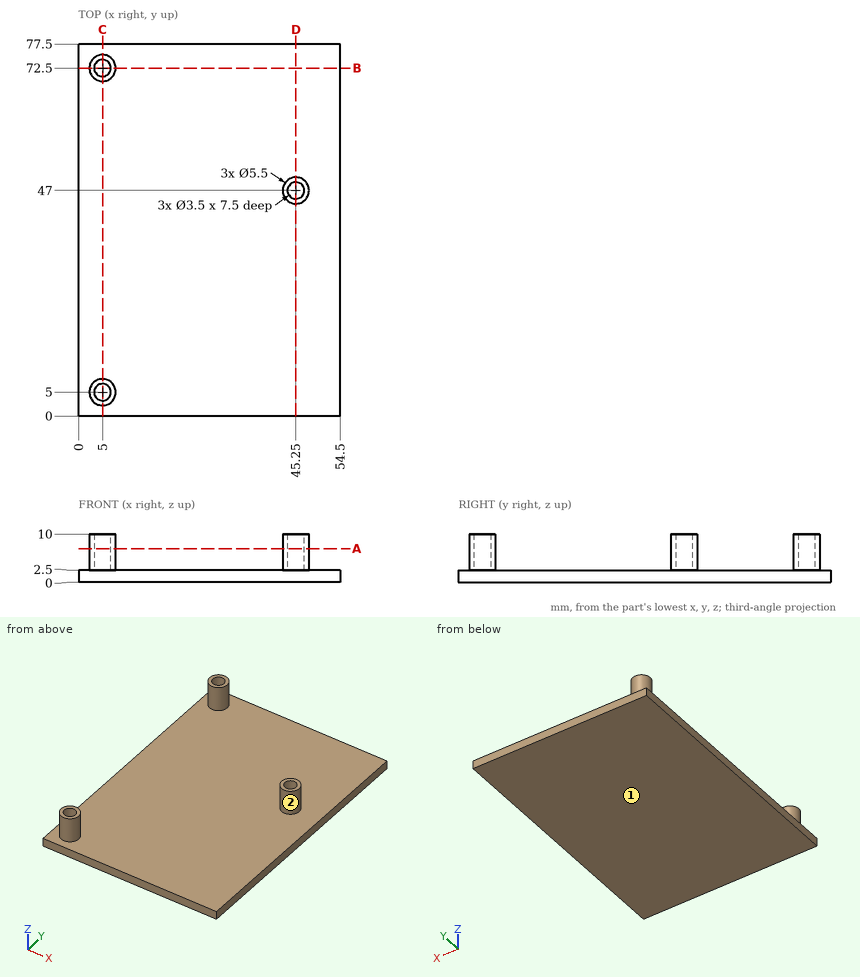
Geometry check sheet. Reference: drawing and pictorial views, mm from the part's lowest x, y, z. A direction names the side the tool comes from. Coordinates: 2 decimals unless noted, no trailing zeros. Write each loop counter-clockwise with the first axis right and the second up, starting at its lowest first coordinate (ties: lowest second). Pieces come first, ordered by that corner, then holes. Notation, with made-up numbers: (-12, 65) -> (12, 65) arc R19 cw to (12, 72) -> close; hole circle Ø10 at (1.5, -6.5). An arc over 180 degrees is marked (long way). Use a Markdown table: item, result.
1. Sectioned sample at A-A (z = 7). Enter the section's corners in (x, y).
Reported:
| item | result |
|---|---|
| outline | circle Ø5.5 at (5, 5); circle Ø5.5 at (5, 72.5); circle Ø5.5 at (45.25, 47); hole circle Ø3.5 at (5, 5); hole circle Ø3.5 at (5, 72.5); hole circle Ø3.5 at (45.25, 47) |
2. Sectioned sample at C-C (x = 5). Enter the section's corners in (y, z).
Reported:
| item | result |
|---|---|
| outline | (0, 0) -> (77.5, 0) -> (77.5, 2.5) -> (75.25, 2.5) -> (75.25, 10) -> (74.25, 10) -> (74.25, 2.5) -> (70.75, 2.5) -> (70.75, 10) -> (69.75, 10) -> (69.75, 2.5) -> (7.75, 2.5) -> (7.75, 10) -> (6.75, 10) -> (6.75, 2.5) -> (3.25, 2.5) -> (3.25, 10) -> (2.25, 10) -> (2.25, 2.5) -> (0, 2.5) -> close |
3. Tool access check on the marked faces 1 and 2. Record the directions out of +Z, -Z, +X, -X, +Y, -Y that give a thin tool (end or side, any length) a straight path to the whole face; none if there is none.
Reported:
| item | result |
|---|---|
| face 1 | -Z, +X, -X, +Y, -Y |
| face 2 | +Z |
4. Sectioned sample at D-D (x = 45.25). Enter the section's corners in (y, z).
Reported:
| item | result |
|---|---|
| outline | (0, 0) -> (77.5, 0) -> (77.5, 2.5) -> (49.75, 2.5) -> (49.75, 10) -> (48.75, 10) -> (48.75, 2.5) -> (45.25, 2.5) -> (45.25, 10) -> (44.25, 10) -> (44.25, 2.5) -> (0, 2.5) -> close |
5. Scan lines: line 1 along Y through (x, z) = (5, 8.5); line 2 along Y through (x, z) = (45.25, 6.75); line 3 along Z through (x, y) = (21, 43.5). Record each from-to range of solid material in increasing order.
Reported:
| item | result |
|---|---|
| line 1 | y = 2.25 to 3.25, 6.75 to 7.75, 69.75 to 70.75, 74.25 to 75.25 |
| line 2 | y = 44.25 to 45.25, 48.75 to 49.75 |
| line 3 | z = 0 to 2.5 |
6. Sectioned sample at B-B (y = 72.5). Enter the section's corners in (x, z).
Reported:
| item | result |
|---|---|
| outline | (0, 0) -> (54.5, 0) -> (54.5, 2.5) -> (7.75, 2.5) -> (7.75, 10) -> (6.75, 10) -> (6.75, 2.5) -> (3.25, 2.5) -> (3.25, 10) -> (2.25, 10) -> (2.25, 2.5) -> (0, 2.5) -> close |
7. Go/stop test with flat-tipped pins: pin 1 Ø5 at (x, y) = (13, 53) entering from +Z; pin 2 Ø1.5 at (x, z) = (7, 5.5) entering from +Y. Record where each tip stops, or that it passes through.
Reported:
| item | result |
|---|---|
| pin 1 | stops at z = 2.5 |
| pin 2 | stops at y = 74.95 |
